from build123d import *

# Parameters (mm, degrees)
SKETCH2_W           = 50.8
SKETCH2_H           = 660.4
BOSS_EXTRUDE1_DEPTH = 50.8
SKETCH5_W           = 50.8
SKETCH5_H           = 50.8
CUT_EXTRUDE1_DEPTH  = 12.7
SKETCH6_W           = 50.8
SKETCH6_H           = 50.8
CUT_EXTRUDE2_DEPTH  = 12.7
SKETCH10_W          = 50.8
SKETCH10_H          = 50.8
CUT_EXTRUDE3_DEPTH  = 12.7
SKETCH11_W          = 50.8
SKETCH11_H          = 50.8
CUT_EXTRUDE4_DEPTH  = 12.7
SKETCH12_R          = 8
CUT_EXTRUDE5_DEPTH  = 16
SKETCH13_R          = 8
CUT_EXTRUDE6_DEPTH  = 16
SKETCH14_R          = 8
CUT_EXTRUDE7_DEPTH  = 16
SKETCH15_R          = 8
CUT_EXTRUDE8_DEPTH  = 16


with BuildPart() as part:
    # Sketch2 → Boss-Extrude1 (new body)
    with BuildSketch(Plane.XY):
        Rectangle(SKETCH2_W, SKETCH2_H)
    extrude(amount=BOSS_EXTRUDE1_DEPTH)

    # Sketch5 → Cut-Extrude1 (cut)
    with BuildSketch(Plane.XY.offset(50.8)):
        with Locations((0, 203.2)):
            Rectangle(SKETCH5_W, SKETCH5_H)
    extrude(amount=-CUT_EXTRUDE1_DEPTH, mode=Mode.SUBTRACT)

    # Sketch6 → Cut-Extrude2 (cut)
    with BuildSketch(Plane(origin=(25.4, 0, 0), x_dir=(0, 0, -1), z_dir=(1, 0, 0))):
        with Locations((-25.4, 203.2)):
            Rectangle(SKETCH6_W, SKETCH6_H)
    extrude(amount=-CUT_EXTRUDE2_DEPTH, mode=Mode.SUBTRACT)

    # Sketch10 → Cut-Extrude3 (cut)
    with BuildSketch(Plane.XY.offset(50.8)):
        with Locations((0, -203.2)):
            Rectangle(SKETCH10_W, SKETCH10_H)
    extrude(amount=-CUT_EXTRUDE3_DEPTH, mode=Mode.SUBTRACT)

    # Sketch11 → Cut-Extrude4 (cut)
    with BuildSketch(Plane(origin=(25.4, 0, 0), x_dir=(0, 0, -1), z_dir=(1, 0, 0))):
        with Locations((-25.4, -203.2)):
            Rectangle(SKETCH11_W, SKETCH11_H)
    extrude(amount=-CUT_EXTRUDE4_DEPTH, mode=Mode.SUBTRACT)

    # Sketch12 → Cut-Extrude5 (cut)
    with BuildSketch(Plane(origin=(0, 0, 0), x_dir=(-1, 0, 0), z_dir=(0, 0, -1))):
        with Locations((0, 304.8)):
            Circle(SKETCH12_R)
    extrude(amount=-CUT_EXTRUDE5_DEPTH, mode=Mode.SUBTRACT)

    # Sketch13 → Cut-Extrude6 (cut)
    with BuildSketch(Plane.ZY.offset(25.4)):
        with Locations((25.4, 304.8)):
            Circle(SKETCH13_R)
    extrude(amount=-CUT_EXTRUDE6_DEPTH, mode=Mode.SUBTRACT)

    # Sketch14 → Cut-Extrude7 (cut)
    with BuildSketch(Plane(origin=(0, 0, 0), x_dir=(-1, 0, 0), z_dir=(0, 0, -1))):
        with Locations((0, -304.8)):
            Circle(SKETCH14_R)
    extrude(amount=-CUT_EXTRUDE7_DEPTH, mode=Mode.SUBTRACT)

    # Sketch15 → Cut-Extrude8 (cut)
    with BuildSketch(Plane.ZY.offset(25.4)):
        with Locations((25.4, -304.8)):
            Circle(SKETCH15_R)
    extrude(amount=-CUT_EXTRUDE8_DEPTH, mode=Mode.SUBTRACT)


solid = part.part
Geometry: final body of the model. Coordinates: model frame, mm. A direction names the side the tool comes from. Give positions to 0.01 mm unless a question says otherwise; leave off trailing zeros. Loops run counter-clockwise (first coordinate to the right, second up) from the corner with the lowest first, then second, coordinate; pieces in that order, holes last. Notation, with made-up numbers: M -0.75,8 L 41.25,8 A14 ccw 41.25,17 Z; hole C 66.5,6.5 d1. An arc over 180 degrees is marked long. Put each result on its own line as item: value. Start each with the question number.
1) Ray query, line 1 along Y through (x, z) = (7.5, 45); line 2 along Y through (x, z) = (0, 10.5); line 3 along X through (y, z) = (-304, 8). Return the intervals inside material, ascending.
2) Cut plane C-C (y = -304.8). Output: boundary loops of the cut face in (x, z).
3) Pull-direction query (X, two-part tool) for faces 1 (the flat face through (0, -279, 50.8)), 2 (the flat face through (25.4, 279, 25)), 3 (the flat face through (0, -305, 16)); classes: pulls with the +X half, pulls with the -X half, needs draft (parallel to the pull), parting line crosses it, or undercut.
4) Cut plane B-B (z = 25.4). Output: boundary loops of the cut face in (x, y).
5) Cut plane A-A (x = -17). Output: boundary loops of the cut face in (y, z), then the cut area to 3 significant figures.
6) Cut plane D-D (y = -202.5). Output: boundary loops of the cut face in (x, z).
7) Contact query for flat-ended pins moving along their axis: pin 1 (11.5 mm diameter, centred on x = -4, y = 194.5, fed in from +Z); pin 2 (11.5 mm diameter, centred on y = 209, z = 15, fed in from +X); pin 3 (5 mm diameter, centred on y = -303, z = 27.5, fed in from -X). Output: stop coordinate, or through.
8) Access query for faces 4 (the flat face through (0, 305, 16)), 5 (the flat face through (-7, 204, 38.1)), 6 (the flat face through (-9.4, -305, 25)), 7 (the flat face through (0, 5, 0)), 8 (the flat face through (11, 177.8, 43)). Directions: +Z, -Z, +X, -X, +Y, -Y. A direction counts if a zero-diameter tool reaches every point of the face in a straight line with its end or side. Return the directions, or none.
Verdict:
1. line 1: -330.2 to -228.6, -177.8 to 177.8, 228.6 to 330.2
1. line 2: -330.2 to -312.8, -296.8 to 296.8, 312.8 to 330.2
1. line 3: -25.4 to -7.96, 7.96 to 25.4
2. outline: M -25.4,0 L -8,0 L -8,16 L 8,16 L 8,0 L 25.4,0 L 25.4,50.8 L -25.4,50.8 L -25.4,33.4 L -9.4,33.4 L -9.4,17.4 L -25.4,17.4 Z
3. face 1: needs draft
3. face 2: pulls with the +X half
3. face 3: undercut
4. outline: M -25.4,-330.2 L 25.4,-330.2 L 25.4,-228.6 L 12.7,-228.6 L 12.7,-177.8 L 25.4,-177.8 L 25.4,177.8 L 12.7,177.8 L 12.7,228.6 L 25.4,228.6 L 25.4,330.2 L -25.4,330.2 L -25.4,312.8 L -9.4,312.8 L -9.4,296.8 L -25.4,296.8 L -25.4,-296.8 L -9.4,-296.8 L -9.4,-312.8 L -25.4,-312.8 Z
5. outline: M -330.2,0 L 330.2,0 L 330.2,50.8 L 228.6,50.8 L 228.6,38.1 L 177.8,38.1 L 177.8,50.8 L -177.8,50.8 L -177.8,38.1 L -228.6,38.1 L -228.6,50.8 L -330.2,50.8 Z; hole C -304.8,25.4 d16; hole C 304.8,25.4 d16
5. area: 31,900 mm2
6. outline: M -25.4,0 L 12.7,0 L 12.7,38.1 L -25.4,38.1 Z
7. pin 1: z = 38.1
7. pin 2: x = 12.7
7. pin 3: x = -9.4
8. face 4: -Z
8. face 5: +Z, +X, -X
8. face 6: -X
8. face 7: -Z, +X, -X, +Y, -Y
8. face 8: +Z, +X
